Part model, mm, in its own coordinate system. A direction names the side the tool comes from. Round coordinates to 2 decimals unless told otherwise and drop trailing zeros. Loops run counter-clockwise (first coordinate to the right, second up) from the corner with the lowest first, then second, coordinate; pieces in that order, holes last. Notation, with made-up numbers: (44, -13) - (61, -13) arc R27 cw to (61, 8) - close; hole circle Ø7 at (-13.5, 4). An arc over 180 degrees is marked (long way). Put each result on its own line as item: value.
from build123d import *

# Parameters (mm, degrees)
F0_W     = 60.7175044715
F0_H     = 55.9188649058
F0_R     = 7.6059383026
F1_DEPTH = 60
F2_R     = 14.7535326744
F3_DEPTH = 2
F4_R     = 7.5183585286
F6_DEPTH = 2
F5_R     = 7.6263318458
F7_DEPTH = 2


with BuildPart() as f1:
    # F0 (on Front) → F1 (new body)
    with BuildSketch(Plane.XZ):
        with Locations((-30.3587522358, 27.9594324529)):
            Rectangle(F0_W, F0_H)
        with Locations((-31.1422031373, 29.4773690403)):
            Circle(F0_R, mode=Mode.SUBTRACT)
        with Locations((-31.1422031373, 29.4773690403)):
            Circle(F0_R)
    extrude(amount=F1_DEPTH)

    # F2 (on face) → F3 (join)
    with BuildSketch(Plane(origin=(-60.7175044715, 0, 0), x_dir=(0, -1, 0), z_dir=(-1, 0, 0))):
        with Locations((28.531210497, 28.0492659658)):
            Circle(F2_R)
    extrude(amount=F3_DEPTH)

    # F4 (on face) → F6 (join)
    with BuildSketch(Plane.XY.offset(55.9188649058)):
        with Locations((-40.4834784567, -29.5914951712)):
            Circle(F4_R)
    extrude(amount=F6_DEPTH)

    # F5 (on face) → F7 (join)
    with BuildSketch(Plane.XY.offset(55.9188649058)):
        with Locations((-21.5911883861, -29.3987151235)):
            Circle(F5_R)
    extrude(amount=F7_DEPTH)


solid = f1.part
1. Band-saw the part on A-A (x = -35.5). List the corners of the cut face in (y, z), plus the area to 3 significant figures.
A:
outline: (-60, 0) - (0, 0) - (0, 55.92) - (-23.96, 55.92) - (-23.96, 57.92) - (-35.22, 57.92) - (-35.22, 55.92) - (-60, 55.92) - close
area: 3,380 mm²
2. Tool access for faces 1 (the cylindrical face through (-61.704, -25.333, 13.647)), 2 (the cylindrical face through (-36.442, -23.252, 56.905)), 3 (the flat face through (-31, -60, 28)): list every direction of +Z, -Z, +X, -X, +Y, -Y with a clear straight run to the whole face (end or side of a thin tool).
A:
face 1: -X
face 2: +Z
face 3: +Z, -Z, +X, -X, -Y
3. Band-saw the part on D-D (x = -7). List the corners of the cut face in (y, z), plus the area to 3 significant figures.
A:
outline: (-60, 0) - (0, 0) - (0, 55.92) - (-60, 55.92) - close
area: 3,360 mm²
4. Pin check, flat tips, straight feed: P1, Ø10, axis at x = -22.5, y = -43.5, coming from the +Z side; P2, Ø8, axis at x = -54.5, y = -47, coming from the -Z side; P3, Ø2, axis at y = -7, z = 22, coming from the -X side. Stop position of each tip, or through.
A:
P1: stops at z = 55.92
P2: stops at z = 0
P3: stops at x = -60.72
5. Band-saw the part on C-C (y = -54). List the corners of the cut face in (x, z).
A:
outline: (-60.72, 0) - (0, 0) - (0, 55.92) - (-60.72, 55.92) - close
6. Band-saw the part on B-B (z = 20). List the corners of the cut face in (x, y).
A:
outline: (-62.72, -40.9) - (-60.72, -40.9) - (-60.72, -60) - (0, -60) - (0, 0) - (-60.72, 0) - (-60.72, -16.17) - (-62.72, -16.17) - close
7. Probe line 1 along Z through (x, y) = (-7, -23.5); line 2 along X through (y, z) = (-46, 45.5). List the from-to ranges inside material, lowest first. Write a range as [from, to].
A:
line 1: z = [0, 55.92]
line 2: x = [-60.72, 0]
8. Two-plate mould, pull along X, no slides. Class faces 4 (the flat face through (-31, 0, 28)), 5 (the flat face through (-60.718, -36, 15)), 6 (the cylindrical face through (-22.584, -21.837, 56.905)): pulls with the +X half, pulls with the -X half, needs draft (parallel to the pull), parting line crosses it, or undercut.
A:
face 4: needs draft
face 5: pulls with the -X half
face 6: undercut
